For this review, take the finished solid that the model builds, in its own axes (mm). A direction names the side the tool comes from. Coordinates: 2 decimals unless noted, no trailing zeros. Write each loop counter-clockwise with the first axis right and the second up, starting at its lowest first coordinate (ties: lowest second). Pieces come first, ordered by that corner, then holes.
```python
from build123d import *

# Parameters (mm, degrees)
SKETCH1_W           = 24.2
SKETCH1_H           = 64
BOSS_EXTRUDE1_DEPTH = 1.5
SKETCH2_R           = 2.2
CUT_EXTRUDE1_DEPTH  = 35.244123583
SKETCH4_W           = 24.2
SKETCH4_H           = 40
BOSS_EXTRUDE2_DEPTH = 1.5
SKETCH5_R           = 3.937
CUT_EXTRUDE2_DEPTH  = 76.184173867
FILLET1_R           = 5


with BuildPart() as part:
    # Sketch1 → Boss-Extrude1 (new body)
    with BuildSketch(Plane.XY):
        Rectangle(SKETCH1_W, SKETCH1_H)
    extrude(amount=BOSS_EXTRUDE1_DEPTH)

    # Sketch2 → Cut-Extrude1 (cut, through all)
    with BuildSketch(Plane.XY.offset(1.5)):
        with Locations((0, -26.8)):
            Circle(SKETCH2_R)
    extrude(amount=-CUT_EXTRUDE1_DEPTH, mode=Mode.SUBTRACT)

    # Sketch4 → Boss-Extrude2 (add)
    with BuildSketch(Plane(origin=(0, 32, 0), x_dir=(1, 0, 0), z_dir=(0, 1, 0))):
        with Locations((0, 20)):
            Rectangle(SKETCH4_W, SKETCH4_H)
    extrude(amount=-BOSS_EXTRUDE2_DEPTH)

    # Sketch5 → Cut-Extrude2 (cut, through all)
    with BuildSketch(Plane.XZ.offset(-30.5)):
        with Locations(Location((0, -20, 0), (0, 0, 270))):
            Circle(SKETCH5_R)
    extrude(amount=-CUT_EXTRUDE2_DEPTH, mode=Mode.SUBTRACT)

    # Fillet1
    fillet1_edges = [part.edges().sort_by_distance(p)[0] for p in [
        (0, 30.5, 0),
    ]]
    fillet(fillet1_edges, radius=FILLET1_R)


solid = part.part
```
Q1. For probe 1 along X at (y, z) = (31, -20); probe 2 along Y at (x, z) = (0, 1.15); probe 3 along Y at (x, z) = (0.75, -29), list the stretches that pass through material, from the lowest coordinate up.
Ans:
probe 1: x = -12.1 to -3.94, 3.94 to 12.1
probe 2: y = -32 to -29, -24.6 to 32
probe 3: y = 30.5 to 32
Q2. Tool access review of faces 1 (the flat face through (12.1, 14, 1)), 2 (the flat face through (0, -3, 0)): name each direction out of +Z, -Z, +X, -X, +Y, -Y from which nothing blocks a thin tool from reaching the whole face with its end or side.
Ans:
face 1: +Z, -Z, +X, +Y, -Y
face 2: -Z, +X, -X, -Y
Q3. Draft analysis for pull direction Y (two halves, no side actions). For faces 3 (the flat face through (0, 0, 1.5)), 4 (the flat face through (-0.2, 32, -24.2)), 5 (the flat face through (0, -32, 1)), 6 (the cylindrical face through (1.02, -28.75, 0.76)), state which applies: +Y half, -Y half, draft (parallel to the pull), parting line (faces both ways), or undercut.
Ans:
face 3: draft
face 4: +Y half
face 5: -Y half
face 6: undercut
Q4. Add section B-B (y = -26.8). State the section outline as (x, z) points.
Ans:
outline: (-12.1, 0) - (-2.2, 0) - (-2.2, 1.5) - (-12.1, 1.5) - close; (2.2, 0) - (12.1, 0) - (12.1, 1.5) - (2.2, 1.5) - close
Q5. Add section D-D (x = -7.75). State the section outline as (y, z) points.
Ans:
outline: (-32, 0) - (25.5, 0) arc R5 cw to (30.5, -5) - (30.5, -40) - (32, -40) - (32, 1.5) - (-32, 1.5) - close
Q6. Add section A-A (x = 0). State the section outline as (y, z) points, then the cut area to 3 significant figures.
Ans:
outline: (-32, 0) - (-29, 0) - (-29, 1.5) - (-32, 1.5) - close; (-24.6, 0) - (25.5, 0) arc R5 cw to (30.5, -5) - (30.5, -16.06) - (32, -16.06) - (32, 1.5) - (-24.6, 1.5) - close; (30.5, -40) - (32, -40) - (32, -23.94) - (30.5, -23.94) - close
area: 143 mm2
Q7. Clearance check with flat-ended pins moving along their axes: pin 1 Ø7.5 at (x, y) = (-2.5, -4.5) entering from -Z; pin 2 Ø12 at (x, z) = (0.5, -28) entering from -Y. State where each tip first meets the part, or that it passes through.
Ans:
pin 1: stops at z = 0
pin 2: stops at y = 30.5
Q8. Add section C-C (z = -20). State the section outline as (x, y) points, then the cut area to 3 significant figures.
Ans:
outline: (-12.1, 30.5) - (-3.94, 30.5) - (-3.94, 32) - (-12.1, 32) - close; (3.94, 30.5) - (12.1, 30.5) - (12.1, 32) - (3.94, 32) - close
area: 24.5 mm2
